Design review of the part built by this model. Coordinates are the model's own, in mm. Round coordinates to 2 decimals unless told otherwise and drop trailing zeros. Write each loop counter-clockwise with the first axis right and the second up, starting at its lowest first coordinate (ties: lowest second). Pieces come first, ordered by that corner, then holes. Notation, with made-up numbers: (-28.5, 50.25) - (-5.5, 50.25) arc R38 ccw to (-5.5, 88.25) - close; hole circle Ø1 at (-8.5, 62.25). An arc over 180 degrees is marked (long way). Use one line per item in the form item = value.
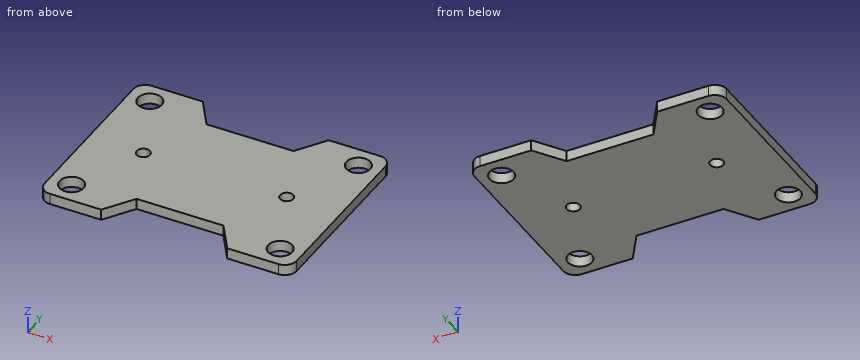
```python
from build123d import *

# Parameters (mm, degrees)
SKETCH1_R           = 2.75
SKETCH1_R_2         = 1.52
BOSS_EXTRUDE1_DEPTH = 2.5
FILLET1_R           = 2.75


with BuildPart() as part:
    # Sketch1 → Boss-Extrude1 (new body)
    with BuildSketch(Plane.XY):
        Polygon((14, 1.75), (34, 1.75), (38.5, -5), (53, -5), (53, 38.5), (38.5, 38.5), (34, 31.75), (14, 31.75), (9.5, 38.5), (-5, 38.5), (-5, -5), (9.5, -5), align=None)
        with Locations((0, 33.5)):
            Circle(SKETCH1_R, mode=Mode.SUBTRACT)
        Circle(SKETCH1_R, mode=Mode.SUBTRACT)
        with Locations((48, 0)):
            Circle(SKETCH1_R, mode=Mode.SUBTRACT)
        with Locations((40.5, 16.75)):
            Circle(SKETCH1_R_2, mode=Mode.SUBTRACT)
        with Locations((7.5, 16.75)):
            Circle(SKETCH1_R_2, mode=Mode.SUBTRACT)
        with Locations((48, 33.5)):
            Circle(SKETCH1_R, mode=Mode.SUBTRACT)
    extrude(amount=BOSS_EXTRUDE1_DEPTH)

    # Fillet1
    fillet1_edges = [part.edges().sort_by_distance(p)[0] for p in [
        (53, -5, 1.25),
        (-5, -5, 1.25),
        (-5, 38.5, 1.25),
        (53, 38.5, 1.25),
    ]]
    fillet(fillet1_edges, radius=FILLET1_R)


solid = part.part
```
Q1. For P1, Ø6.5, axis at x = 0, y = 33.5, coming from the -Z side; P2, Ø1.2, axis at x = 22.5, z = 0.5, coming from the +Y side, all flat-tipped, find the tip position at first contact; note any pin that passes through.
Calculated:
P1 = 0
P2 = 31.75
Q2. To check wall thickness, follow line 1 along Y through (x, z) = (0, 1.05); line 2 along Y through (x, z) = (49, 1.4); line 3 along Y through (x, z) = (40.5, 1.35). State the ranges of each line that lie inside material, in increasing order. Write a range as from..to.
Calculated:
line_1 = -5..-2.75, 2.75..30.75, 36.25..38.5
line_2 = -5..-2.56, 2.56..30.94, 36.06..38.5
line_3 = -5..15.23, 18.27..38.5
Q3. We need section C-C on z = 1.2. Write out the cut boundary in (x, y), then the cut area to 3 significant figures.
Calculated:
outline = (-5, -2.25) arc R2.75 ccw to (-2.25, -5) - (9.5, -5) - (14, 1.75) - (34, 1.75) - (38.5, -5) - (50.25, -5) arc R2.75 ccw to (53, -2.25) - (53, 35.75) arc R2.75 ccw to (50.25, 38.5) - (38.5, 38.5) - (34, 31.75) - (14, 31.75) - (9.5, 38.5) - (-2.25, 38.5) arc R2.75 ccw to (-5, 35.75) - close; hole circle Ø5.5 at (0, 0); hole circle Ø5.5 at (0, 33.5); hole circle Ø3.04 at (7.5, 16.75); hole circle Ø3.04 at (40.5, 16.75); hole circle Ø5.5 at (48, 0); hole circle Ø5.5 at (48, 33.5)
area = 2,080 mm2
Q4. We need section D-D on x = 40.5. Write out the cut boundary in (y, z), then the cut area to 3 significant figures.
Calculated:
outline = (-5, 0) - (15.23, 0) - (15.23, 2.5) - (-5, 2.5) - close; (18.27, 0) - (38.5, 0) - (38.5, 2.5) - (18.27, 2.5) - close
area = 101 mm2
Q5. We need section B-B on x = 48. Write out the cut boundary in (y, z), then the cut area to 4 significant figures.
Calculated:
outline = (-5, 0) - (-2.75, 0) - (-2.75, 2.5) - (-5, 2.5) - close; (2.75, 0) - (30.75, 0) - (30.75, 2.5) - (2.75, 2.5) - close; (36.25, 0) - (38.5, 0) - (38.5, 2.5) - (36.25, 2.5) - close
area = 81.25 mm2
Q6. We need section A-A on y = 16.75. Write out the cut boundary in (x, z).
Calculated:
outline = (-5, 0) - (5.98, 0) - (5.98, 2.5) - (-5, 2.5) - close; (9.02, 0) - (38.98, 0) - (38.98, 2.5) - (9.02, 2.5) - close; (42.02, 0) - (53, 0) - (53, 2.5) - (42.02, 2.5) - close
